Answer from the drawing. Dimensions are ordinates in mm from the lowest x, y and z of the part. Coordinates: 2 decimals unless noted, no trailing zeros. Loops run counter-clockwise (first coordinate to the right, second up) from the corner with the lowest first, then second, coordinate; pieces in that order, holes last.
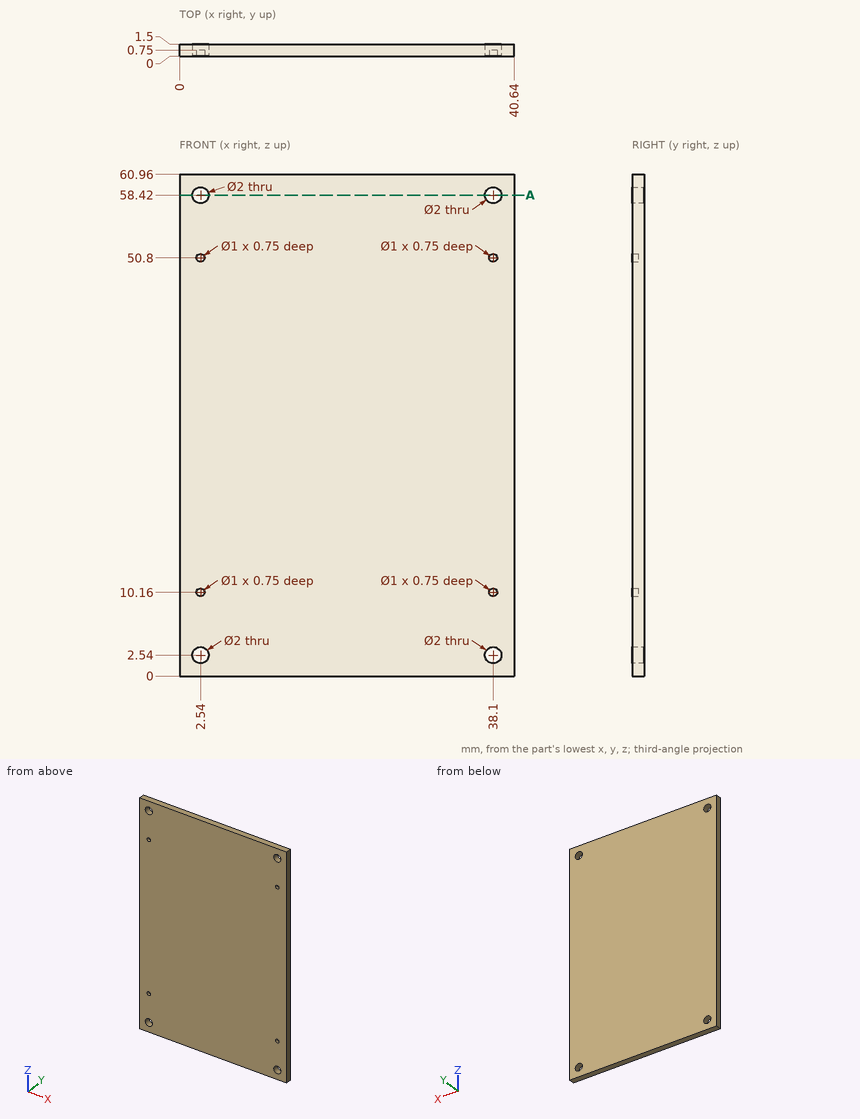
Item 1: A cutting plane is placed at A-A on z = 58.42. Determine the outline of the cut face in (x, y), then the cut area to 3 significant figures.
Numbers:
outline: (0, 0) - (1.54, 0) - (1.54, 1.5) - (0, 1.5) - close; (3.54, 0) - (37.1, 0) - (37.1, 1.5) - (3.54, 1.5) - close; (39.1, 0) - (40.64, 0) - (40.64, 1.5) - (39.1, 1.5) - close
area: 55.0 mm2
Item 2: Given pin 1 (0.5 mm diameter, centred on x = 2.5, z = 10, fed in from -Y), flat-ended and moving along its own axis, determine where the tip first touches the part or whether it passes through.
Numbers:
pin 1: stops at y = 0.75
Item 3: Find the intervals of material crossed by line 1 along X through (y, z) = (0.4, 50.8); line 2 along X through (y, z) = (0.85, 58.42); line 3 along Z through (x, y) = (38.5, 0.3), in increasing order.
Numbers:
line 1: x = 0 to 2.04, 3.04 to 37.6, 38.6 to 40.64
line 2: x = 0 to 1.54, 3.54 to 37.1, 39.1 to 40.64
line 3: z = 0 to 1.62, 3.46 to 9.86, 10.46 to 50.5, 51.1 to 57.5, 59.34 to 60.96
